Input: part model. Units: mm. Frame: model coordinates. Face numbers are marked on the shaded views. Coordinates: 2 decimals unless noted, no trailing zeros. Loops run counter-clockwise (first coordinate to the right, second up) from the corner with the lowest first, then second, coordinate; pieces in that order, holes last. Notation, with made-up numbers: (55.25, -24) -> (74.25, -24) arc R15 cw to (74.25, -20) -> close; hole circle Ø9 at (-34, 36.5). An arc over 180 degrees is marked (long way). Put each result on its own line as item: value. Start each with the question number.
1) Pull-direction query (Y, two-part tool) for the marked faces 1, 2 and 3; classes: pulls with the +Y half, pulls with the -Y half, needs draft (parallel to the pull), parting line crosses it, or undercut.
2) Cut plane C-C (y = 0). Return the cut outline in (x, z).
3) Cut plane D-D (z = -9.5). Return the cut outline in (x, y), plus the area to 3 significant figures.
4) Cut plane A-A (z = 0). Return the cut outline in (x, y), plus the area to 3 significant figures.
5) Contact query for flat-ended pins moving along their axis: P1, Ø5, axis at y = 1, z = -8, coming from the -X side; P2, Ø2, axis at x = 1.5, y = -8.5, coming from the +Z side. Output: stop coordinate, or through.
6) Material intervals for L1, parallel to Y at x = -16, z = 0; L2, parallel to Y at x = 2, z = 4.25; L3, parallel to Z at x = 27, y = 0, sorted ascending.
7) Cut plane B-B (x = -16.5). Return the cut outline in (y, z), plus the area to 3 significant figures.
from build123d import *

# Parameters (mm, degrees)
F1_R          = 12.7
F2_DEPTH      = 70
F2_DEPTH_BACK = 70
F3_W          = 35.4
F3_H          = 19.7
F4_DEPTH      = 70
F4_DEPTH_BACK = 70


with BuildPart() as f2:
    # F1 (on Right) → F2 (new body, two sides)
    with BuildSketch(Plane.YZ) as f2_sk:
        Circle(F1_R)
    extrude(amount=F2_DEPTH)
    extrude(f2_sk.sketch, amount=-F2_DEPTH_BACK)


with BuildPart() as f4:
    # F3 (on Right) → F4 (new body, two sides)
    with BuildSketch(Plane.YZ) as f4_sk:
        with Locations((0, -3.85)):
            Rectangle(F3_W, F3_H)
    extrude(amount=F4_DEPTH)
    extrude(f4_sk.sketch, amount=-F4_DEPTH_BACK)

    # F5: cut F2
    add(f2.part, mode=Mode.SUBTRACT)


solid = f4.part
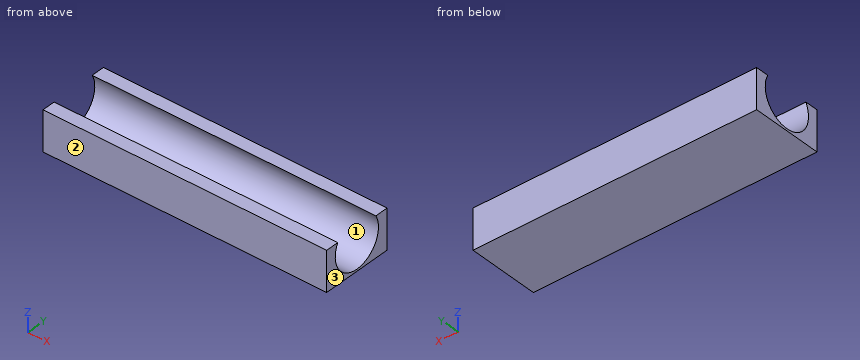
Results found:
1. face 1: undercut
1. face 2: pulls with the -Y half
1. face 3: needs draft
2. outline: (-70, -13.7) -> (70, -13.7) -> (70, -12.7) -> (-70, -12.7) -> close
3. outline: (-70, -17.7) -> (70, -17.7) -> (70, -8.43) -> (-70, -8.43) -> close; (-70, 8.43) -> (70, 8.43) -> (70, 17.7) -> (-70, 17.7) -> close
3. area: 2,600 mm2
4. outline: (-70, -17.7) -> (70, -17.7) -> (70, -12.7) -> (-70, -12.7) -> close; (-70, 12.7) -> (70, 12.7) -> (70, 17.7) -> (-70, 17.7) -> close
4. area: 1,400 mm2
5. P1: passes through
5. P2: stops at z = -8.43
6. L1: y = -17.7 to -12.7, 12.7 to 17.7
6. L2: y = -17.7 to -11.97, 11.97 to 17.7
6. L3: z = -13.7 to -12.7
7. outline: (-17.7, -13.7) -> (17.7, -13.7) -> (17.7, 6) -> (11.19, 6) arc R12.7 cw (long way) to (-11.19, 6) -> (-17.7, 6) -> close
7. area: 298 mm2
